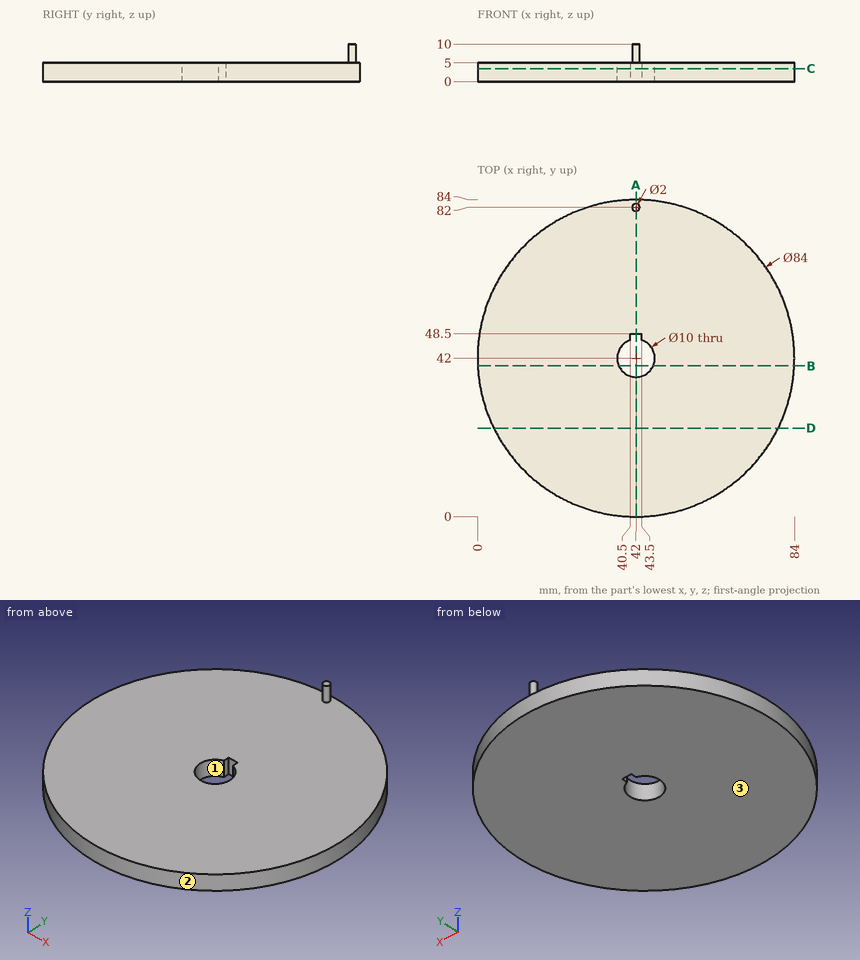
Print and shaded views of the part. All mm, measured from the part's lowest x, y and z. Round coordinates to 2 decimals unless told otherwise and drop trailing zeros. Write each loop counter-clockwise with the first axis right and the second up, starting at its lowest first coordinate (ties: lowest second). Pieces come first, ordered by that corner, then holes.
(1) Mould opens along Y. For the marked faces 1, 2 and 3 say: pulls with the +Y half, pulls with the -Y half, needs draft (parallel to the pull), parting line crosses it, or undercut.
(2) Slice it at A-A, the plane x = 42. Write the cut outline in (y, z).
(3) Slice it at C-C, the plane z = 3.5. Write the cut outline in (x, y), and give its area (3 significant figures).
(4) Slice it at B-B, the plane y = 40. Write the cut outline in (x, z).
(5) Slice it at D-D, the plane y = 23.5. Write the cut outline in (x, z), and give its area (3 significant figures).
(6) Probe line 1 along Y through (x, z) = (42, 2.75); line 2 along Z through (x, y) = (63, 47); line 3 along X through (y, z) = (37.5, 2.75). List the from-to ranges inside material, lowest first.
(7) Drop flat-ended pins along their axis: P1, Ø3, axis at y = 9, z = 7, coming from the +X side; P2, Ø3, axis at y = 72.5, z = 1.5, coming from the +X side; P3, Ø1.4, axis at y = 47.5, z = 1.5, coming from the +X side; P4, Ø1.5, axis at x = 41.5, z = 2, coming from the -Y side. Give the stop position or say it passes through.
From the geometry:
1. face 1: undercut
1. face 2: parting line crosses it
1. face 3: needs draft
2. outline: (0, 0) - (37, 0) - (37, 5) - (0, 5) - close; (48.5, 0) - (84, 0) - (84, 5) - (83, 5) - (83, 10) - (81, 10) - (81, 5) - (48.5, 5) - close
3. outline: circle Ø84 at (42, 42); hole (40.5, 46.77) arc R5 ccw (long way) to (43.5, 46.77) - (43.5, 48.5) - (40.5, 48.5) - close
3. area: 5,460 mm2
4. outline: (0.05, 0) - (37.42, 0) - (37.42, 5) - (0.05, 5) - close; (46.58, 0) - (83.95, 0) - (83.95, 5) - (46.58, 5) - close
5. outline: (4.29, 0) - (79.71, 0) - (79.71, 5) - (4.29, 5) - close
5. area: 377 mm2
6. line 1: y = 0 to 37, 48.5 to 84
6. line 2: z = 0 to 5
6. line 3: x = 0.24 to 39.82, 44.18 to 83.76
7. P1: passes through
7. P2: stops at x = 72.38
7. P3: stops at x = 83.72
7. P4: stops at y = 0
